The model under review builds one solid part; all positions refer to its coordinate system, in mm. A direction names the side the tool comes from. Coordinates: 2 decimals unless noted, no trailing zeros. Write each loop counter-clockwise with the first axis right and the second up, starting at its lowest first coordinate (ties: lowest second). Pieces come first, ordered by that corner, then holes.
Autodesk Inventor part; units mm, degrees
ref_plane "YZ Plane" through (0, 0, 0) normal (1, 0, 0) x (0, 1, 0)
ref_plane "XZ Plane" through (0, 0, 0) normal (0, 1, 0) x (-1, 0, 0)
ref_plane "XY Plane" through (0, 0, 0) normal (0, 0, 1) x (1, 0, 0)
sketch "Skizze1" plane through (0, 0, 0) normal (0, 1, 0) x (-1, 0, 0)
  circle A0 centre (0, 0) radius 8
  circle A1 centre (-8, 0) radius 3
  circle A2 centre (8, 0) radius 3
  line L0 (8, 0) -> (-8, 0)
  dimension "d0" = 16
  dimension "d1" = 6
  dimension "d2" = 6
extrude "Extrusion1" add sketch "Skizze1" along normal blind 1
sketch "Skizze2" plane through (0, 1, 0) normal (0, 1, 0) x (1, 0, 0)
  arc A0 (7.4375, 2.9468) -> (-7.4375, 2.9468) centre (0, 0) ccw
  circle A1 centre (0, 0) radius 5.875
  circle A2 centre (0, 0) radius 4.5
  dimension "d5" = 11.75
  dimension "d6" = 9
extrude "Extrusion2" add sketch "Skizze2" along normal blind 0.5
sketch "Skizze3" plane through (0, 1, 0) normal (0, 1, 0) x (1, 0, 0)
  arc A0 (7.4375, -2.9468) -> (7.4375, 2.9468) centre (8, 0) ccw
  arc A1 (-7.4375, 2.9468) -> (-7.4375, -2.9468) centre (-8, 0) ccw
  circle A2 centre (-8, 0) radius 1.375
  circle A3 centre (8, 0) radius 1.375
  dimension "d9" = 2.75
  dimension "d10" = 2.75
extrude "Extrusion3" cut sketch "Skizze3" against normal up to next
properties part number "top"
Item 1: Take a section at A-A, the plane z = 0. Write out the cut boundary in (x, y) (3 decimals).
Solved:
outline: (-11, 0) - (-9.375, 0) - (-9.375, 1) - (-11, 1) - close; (-6.625, 0) - (6.625, 0) - (6.625, 1) - (5.875, 1) - (5.875, 1.5) - (4.5, 1.5) - (4.5, 1) - (-4.5, 1) - (-4.5, 1.5) - (-5.875, 1.5) - (-5.875, 1) - (-6.625, 1) - close; (9.375, 0) - (11, 0) - (11, 1) - (9.375, 1) - close
Item 2: Mouldability with a two-part tool opening along X and no side actions: class faces 3 (the face through (-0.59, 1.25, 4.46)), 4 (the face through (5.604, 1.246, 1.765)), 5 (the face through (1.713, 1.5, 4.324)), 6 (the face through (-9.374, 0.507, -0.06)) as pulls with the +X half, pulls with the -X half, needs draft (parallel to the pull), parting line crosses it, or undercut.
Solved:
face 3: undercut
face 4: parting line crosses it
face 5: needs draft
face 6: undercut
Item 3: Take a section at C-C, the plane y = 0.5. Count the separate pieces of the cut face and the enclosed holes in it, plus the area to 3 significant figures.
Solved:
separate pieces: 1
enclosed holes: 2
area: 220 mm2
Item 4: Take a section at B-B, the plane x = 8. Write out the cut boundary in (y, z) (3 decimals).
Solved:
outline: (0, -3) - (1, -3) - (1, -1.375) - (0, -1.375) - close; (0, 1.375) - (1, 1.375) - (1, 3) - (0, 3) - close
Item 5: Take a section at D-D, the plane x = 0. Write out the cut boundary in (y, z) (3 decimals), plus the area to 3 significant figures.
Solved:
outline: (0, -8) - (1, -8) - (1, -5.875) - (1.5, -5.875) - (1.5, -4.5) - (1, -4.5) - (1, 4.5) - (1.5, 4.5) - (1.5, 5.875) - (1, 5.875) - (1, 8) - (0, 8) - close
area: 17.4 mm2
Item 6: For pin 1 (8 mm diameter, centred on x = -7.5, z = -1.5, fed in from -Y); pin 2 (1.6 mm diameter, centred on x = 8, z = 0, fed in from +Y), all flat-tipped, find the tip position at first contact; note any pin that passes through.
Solved:
pin 1: stops at y = 0
pin 2: passes through
Item 7: Machinability: for faces 1 (the face through (0, 0, 0)), 2 (the face through (-6, 1, 2)), which of the approach directions +Z, -Z, +X, -X, +Y, -Y give a long, thin tool a straight path to every point of the face, cutting with its end or side? Answer none if there is none.
Solved:
face 1: +Z, -Z, +X, -X, -Y
face 2: +Y
Item 8: To check wall thickness, follow line 1 along Z through (x, y) = (0, 1.25) (3 decimals); line 2 along X through (y, z) = (0.8, -1). State the ranges of each line that lie inside material, in increasing order.
Solved:
line 1: z = -5.875 to -4.5, 4.5 to 5.875
line 2: x = -10.83 to -8.94, -7.06 to 7.06, 8.94 to 10.83
